Input: part model. Units: mm. Frame: model coordinates. Face numbers are marked on the shaded views. A direction names the side the tool comes from. Coordinates: 2 decimals unless noted, no trailing zeros. Order: outer loops, then holes, each group sorted by start corner. A loop starts at its lowest first (then second) coordinate and runs counter-clockwise, first axis right, second up. Notation, with made-up numbers: M 34,75.25 L 84,75.25 A5 cw 84,84.25 Z; hole C 49.5,82.5 d11. An arc over 180 degrees is marked long. Answer in a Markdown table with one row per item.
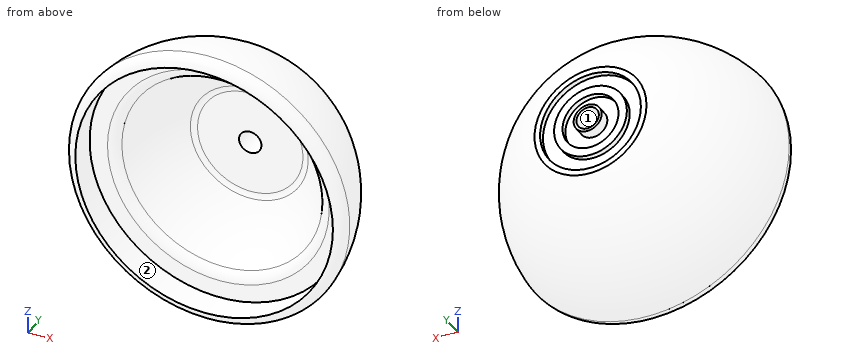
from build123d import *

# Parameters (mm, degrees)
F2_R      = 9
F2_R_2    = 6.5
F3_DEPTH  = 1
F4_R      = 5
F5_DEPTH  = 1
F6_R      = 23
F7_DEPTH  = 5
F8_R      = 2.5
F9_DEPTH  = 2
F10_R     = 2
F11_DEPTH = 25


# Not quite as in the source:
# - a fillet or chamfer that OpenCascade refuses, or shapes differently, is made with other operations: its cross-section is extruded or revolved along the edge and cut away or added


with BuildPart() as f1:
    # F0 (on Top) → F1 (revolve)
    with BuildSketch(Plane.XY):
        with BuildLine():
            ThreePointArc((-30.0702019767, 18.8458363465), (-40.98670264, 9.6260218093), (-45.0702019767, -4.0670421283))
            Line((-45.0702019767, -4.0670421283), (-39.0702019767, -4.0670421283))
            ThreePointArc((-39.0702019767, -4.0670421283), (-36.6683946494, 5.1795788761), (-30.0702019767, 12.0884522931))
            ThreePointArc((-30.0702019767, 12.0884522931), (-25.2685481557, 14.2080008813), (-20.0702019767, 14.9329578717))
            Line((-20.0702019767, 14.9329578717), (-20.0702019767, 18.8458363465))
            Line((-20.0702019767, 18.8458363465), (-30.0702019767, 18.8458363465))
        make_face()
        with BuildLine():
            ThreePointArc((-20.0702019767, 14.9329578717), (-25.2685481557, 14.2080008813), (-30.0702019767, 12.0884522931))
            Line((-30.0702019767, 12.0884522931), (-20.0702019767, 12.0884522931))
            Line((-20.0702019767, 12.0884522931), (-20.0702019767, 14.9329578717))
        make_face()
    revolve(axis=Axis((-20.0702019767, 9.4528388078, 0), (0, 1, 0)))

    # F2 (on face) → F3 (cut)
    with BuildSketch(Plane(origin=(0, 18.8458363465, 0), x_dir=(-1, 0, 0), z_dir=(0, 1, 0))):
        with Locations((20.0702019767, 0)):
            Circle(F2_R)
        with Locations((20.0702019767, 0)):
            Circle(F2_R_2, mode=Mode.SUBTRACT)
    extrude(amount=-F3_DEPTH, mode=Mode.SUBTRACT)

    # F4 (on face) → F5 (cut)
    with BuildSketch(Plane(origin=(0, 18.8458363465, 0), x_dir=(-1, 0, 0), z_dir=(0, 1, 0))):
        with Locations((20.0702019767, 0)):
            Circle(F4_R)
    extrude(amount=-F5_DEPTH, mode=Mode.SUBTRACT)

    # F6 (on face) → F7 (cut)
    with BuildSketch(Plane.XZ.offset(4.0670421283)):
        with Locations((-20.0702019767, 0)):
            Circle(F6_R)
    extrude(amount=-F7_DEPTH, mode=Mode.SUBTRACT)

    # F8 (on face) → F9 (join)
    with BuildSketch(Plane(origin=(0, 17.8458363465, 0), x_dir=(-1, 0, 0), z_dir=(0, 1, 0))):
        with Locations((20.0702019767, 0)):
            Circle(F8_R)
    extrude(amount=F9_DEPTH)

    # F10 (on face) → F11 (cut)
    with BuildSketch(Plane(origin=(0, 19.8458363465, 0), x_dir=(-1, 0, 0), z_dir=(0, 1, 0))):
        with Locations((20.0702019767, 0)):
            Circle(F10_R)
    extrude(amount=-F11_DEPTH, mode=Mode.SUBTRACT)

    # F12: fillet of radius 2 on 3 edges, made by hand

    # F12_s1 → F12_t2 (revolve)
    with BuildSketch(Plane.XY):
        with BuildLine():
            ThreePointArc((-30.5916471957, 11.753804578), (-30.0626140836, 12.0029632711), (-29.4841266463, 12.0884522931))
            Line((-29.4841266463, 12.0884522931), (-30.0702019767, 12.0884522931))
            ThreePointArc((-30.0702019767, 12.0884522931), (-30.3322887889, 11.9232541247), (-30.5916471957, 11.753804578))
        make_face()
    revolve(axis=Axis((-20.0702019767, 12.0884522931, 0), (0, 1, 0)))

    # F12_s3 → F12_t4 (revolve, cut)
    with BuildSketch(Plane.XY):
        with BuildLine():
            ThreePointArc((-44.9756840183, -1.895184795), (-44.4866456176, -3.3879435981), (-43.0702019767, -4.0670421283))
            Line((-43.0702019767, -4.0670421283), (-45.0702019767, -4.0670421283))
            ThreePointArc((-45.0702019767, -4.0670421283), (-45.0465613095, -2.9800856066), (-44.9756840183, -1.895184795))
        make_face()
    revolve(axis=Axis((-20.0702019767, -4.0670421283, 0), (0, 1, 0)), mode=Mode.SUBTRACT)

    # F12_s5 → F12_t6 (revolve, cut)
    with BuildSketch(Plane.XY):
        with BuildLine():
            ThreePointArc((-39.8691918499, 0.9329578717), (-38.7144913115, 1.2999647098), (-37.9835737667, 2.266291205))
            ThreePointArc((-37.9835737667, 2.266291205), (-38.2042977916, 1.6034577592), (-38.4005047565, 0.9329578717))
            Line((-38.4005047565, 0.9329578717), (-39.8691918499, 0.9329578717))
        make_face()
    revolve(axis=Axis((-20.0702019767, 0.9329578717, 0), (0, 1, 0)), mode=Mode.SUBTRACT)


solid = f1.part
1) Material intervals for probe 1 along Z at (x, y) = (-2.5, 10.25); probe 2 along Z at (x, y) = (-26, 5.5); probe 3 along X at (y, z) = (10.25, -0.5), sorted ascending.
Resolved:
| item | result |
|---|---|
| probe 1 | z = -10.55 to 10.55 |
| probe 2 | z = -22.32 to -15.31, 15.31 to 22.32 |
| probe 3 | x = -40.56 to -32.55, -7.59 to 0.42 |
2) Cut plane A-A, the plane y = 11. Output: boundary loops of the cut face in (x, z), and give its area (3 significant figures).
Resolved:
| item | result |
|---|---|
| outline | C -20.07,0 d39.9; hole C -20.07,0 d23.15 |
| area | 829 mm2 |
3) Reachability of the marked faces 1 and 2 from +Z, -Z, +X, -X, +Y, -Y: full face, straight path, thin tool, end or side. Return the list, or none.
Resolved:
| item | result |
|---|---|
| face 1 | +Y, -Y |
| face 2 | -Y |
4) Contact query for flat-ended pins moving along their axis: pin 1 (6 mm diameter, centred on x = -16.5, z = 7, fed in from -Y); pin 2 (10 mm diameter, centred on x = -15, z = 6, fed in from -Y); pin 3 (2 mm diameter, centred on x = -34.5, z = 11, fed in from +Y). Output: stop coordinate, or through.
Resolved:
| item | result |
|---|---|
| pin 1 | stops at y = 11.52 |
| pin 2 | stops at y = 9.92 |
| pin 3 | stops at y = 14.13 |
